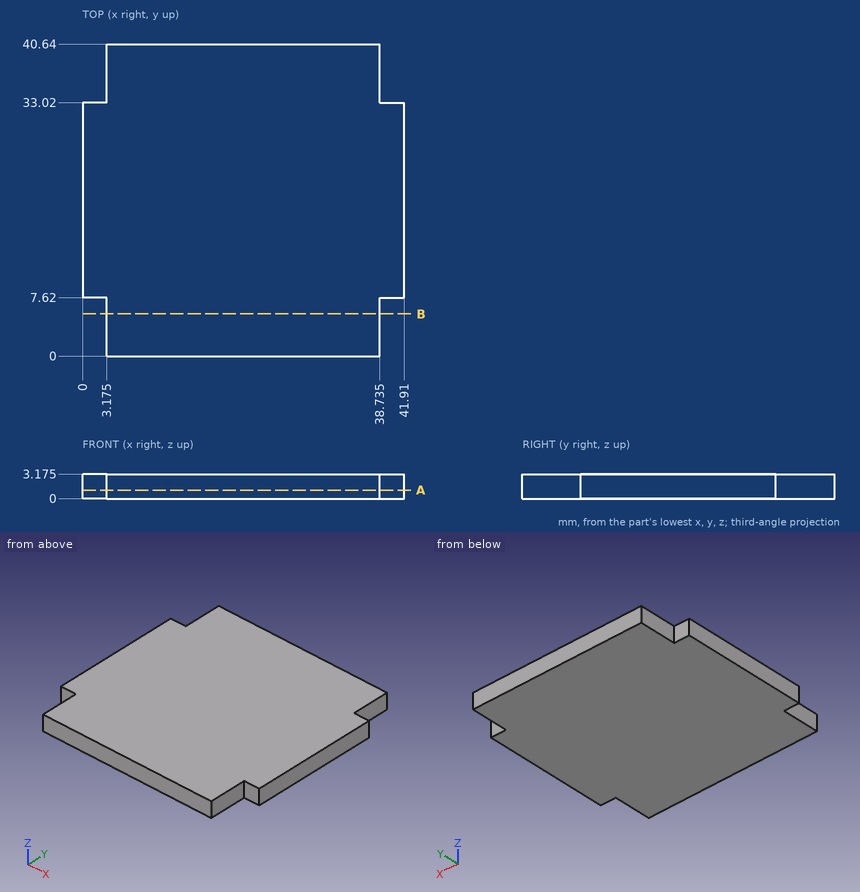
For this review, use the dimensioned drawing (mm, ordinates from the lowest corner) and the shaded views. Round coordinates to 2 decimals unless told otherwise and drop trailing zeros. Write each loop counter-clockwise with the first axis right and the second up, starting at its lowest first coordinate (ties: lowest second). Pieces come first, ordered by that corner, then holes. Notation, with made-up numbers: (-4, 85.5) -> (10, 85.5) arc R20 ccw to (10, 97.5) -> close; hole circle Ø2 at (81, -15). An arc over 180 degrees is marked (long way). One line per item, written item: value. Start each with the question number.
Q1. Add section A-A (z = 1.1). Give the boundary of the cut face in (x, y) (3 decimals).
Q2. Add section B-B (y = 5.5). Give the boundary of the cut face in (x, z) (3 decimals).
Q3. Insertion check: P1, Ø1, axis at y = 37.5, z = 1.5, coming from the -X side (3 decimals); P2, Ø1, axis at y = 36, z = 1, coming from the +X side (3 decimals); P3, Ø1.6, axis at x = 40, z = 2, coming from the -Y side. Each pin has a flat end and moves straight along its axis. Give the tip position at first contact, or say it passes through.
Q4. To check wall thickness, follow probe 1 along X at (y, z) = (5.5, 2.45) (3 decimals); probe 2 along Y at (x, z) = (39.5, 2.25). State the ranges of each line that lie inside material, in increasing order.
Response:
1. outline: (0, 7.62) -> (3.175, 7.62) -> (3.175, 0) -> (38.735, 0) -> (38.735, 7.62) -> (41.91, 7.62) -> (41.91, 33.02) -> (38.735, 33.02) -> (38.735, 40.64) -> (3.175, 40.64) -> (3.175, 33.02) -> (0, 33.02) -> close
2. outline: (3.175, 0) -> (38.735, 0) -> (38.735, 3.175) -> (3.175, 3.175) -> close
3. P1: stops at x = 3.175
3. P2: stops at x = 38.735
3. P3: stops at y = 7.62
4. probe 1: x = 3.175 to 38.735
4. probe 2: y = 7.62 to 33.02
